Input: dimensioned drawing with shaded views. Units: mm. Origin: part minimum x, y, z. A direction names the side the tool comes from. Give positions to 0.01 mm unless a question says otherwise; leave off trailing zeros. Loops run counter-clockwise (first coordinate to the right, second up) from the corner with the lowest first, then second, coordinate; pieces in that order, holes last. Notation, with made-up numbers: (1.5, 1.5) -> (45.5, 1.5) arc R15 cw to (45.5, 18.5) -> close; hole circle Ø10 at (17.25, 58.25). An arc over 180 degrees is marked (long way). Answer as a JSON object with one key per item and string values.
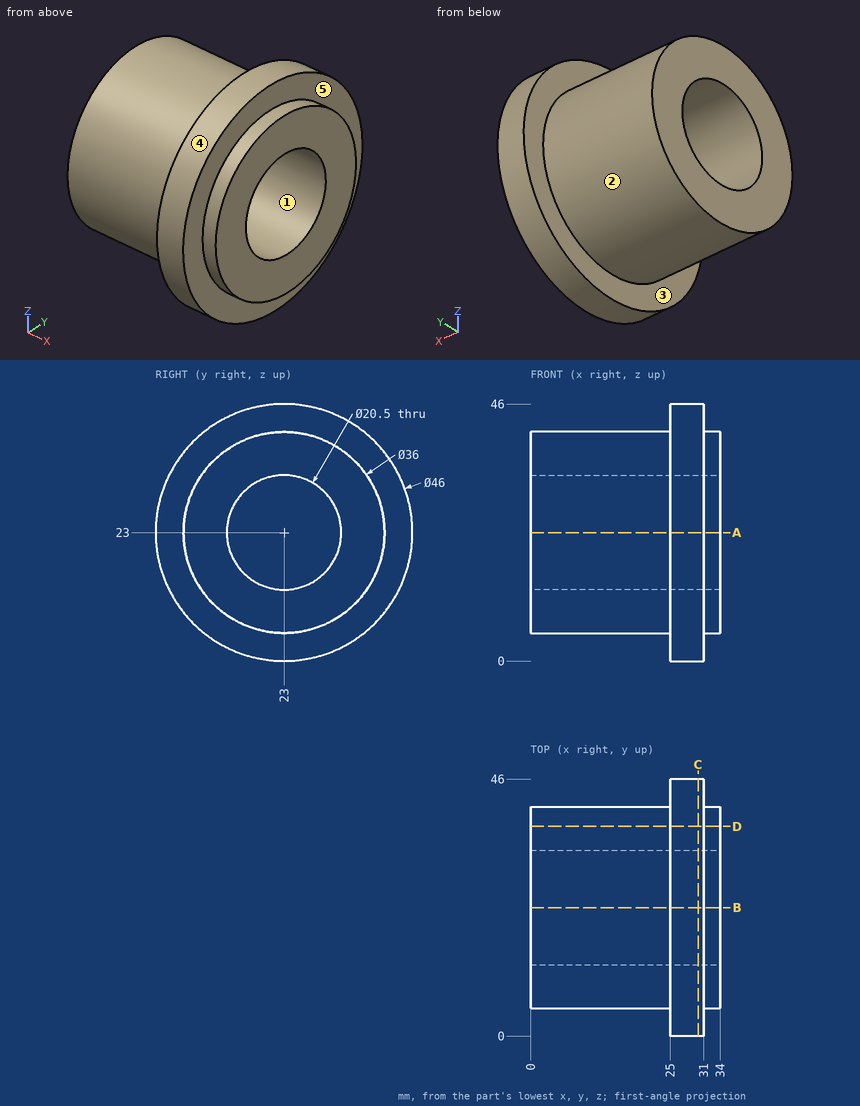
Q1. Pin query (flat end, axial travel): pin 1 (1.5 mm diameter, centred on y = 5.5, z = 14, fed in from -X); pin 2 (4 mm diameter, centred on x = 17.5, z = 20, fed in from -Y); pin 3 (12 mm diameter, centred on x = 24.5, z = 29.5, fed in from +Y); pin 4 (16.5 mm diameter, centred on y = 23, z = 23, fed in from -X). Return the tip coordinate at first contact, or that it passes through.
Evaluation:
{"pin 1": "stops at x = 25", "pin 2": "stops at y = 5.03", "pin 3": "stops at y = 45.99", "pin 4": "passes through"}
Q2. Draft query along Y for the marked faces 1, 2 and 3. Return one class per face: +Y half, -Y half, draft (parallel to the pull), parting line (faces both ways), or undercut.
Evaluation:
{"face 1": "undercut", "face 2": "parting line", "face 3": "draft"}
Q3. Section C-C, the plane x = 30. Return the cut outline in (y, z), then the cut area to 3 significant figures.
Evaluation:
{"outline": "circle Ø46 at (23, 23); hole circle Ø20.5 at (23, 23)", "area": "1,330 mm2"}
Q4. Section D-D, the plane y = 37.5. Return the cut outline in (x, z), then the cut area to 3 significant figures.
Evaluation:
{"outline": "(0, 12.33) -> (25, 12.33) -> (25, 5.15) -> (31, 5.15) -> (31, 12.33) -> (34, 12.33) -> (34, 33.67) -> (31, 33.67) -> (31, 40.85) -> (25, 40.85) -> (25, 33.67) -> (0, 33.67) -> close", "area": "812 mm2"}
Q5. Section A-A, the plane z = 23. Return the cut outline in (x, y), then the cut area to 3 significant figures.
Evaluation:
{"outline": "(0, 5) -> (25, 5) -> (25, 0) -> (31, 0) -> (31, 5) -> (34, 5) -> (34, 12.75) -> (0, 12.75) -> close; (0, 33.25) -> (34, 33.25) -> (34, 41) -> (31, 41) -> (31, 46) -> (25, 46) -> (25, 41) -> (0, 41) -> close", "area": "587 mm2"}
Q6. Ray query, line 1 along Y through (x, z) = (10, 23); line 2 along X through (y, z) = (14.5, 39); line 3 along Y through (x, z) = (26, 23). Return the intervals inside material, ascending.
Evaluation:
{"line 1": "y = 5 to 12.75, 33.25 to 41", "line 2": "x = 25 to 31", "line 3": "y = 0 to 12.75, 33.25 to 46"}
Q7. Access query for the marked faces 4 and 5. Directions: +Z, -Z, +X, -X, +Y, -Y. A direction counts if a zero-diameter tool reaches every point of the face in a straight line with its end or side. Return the directions, or none.
Evaluation:
{"face 4": "+X, -X", "face 5": "+X"}
